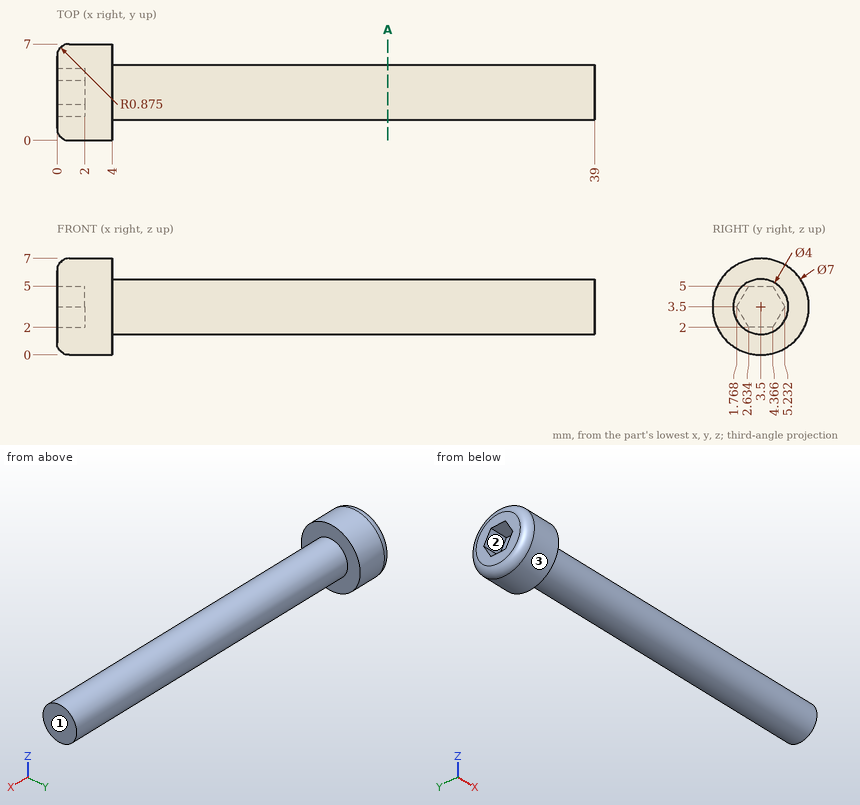
Here's the drawing with two shaded views (mm, measured from the low corner). I have some questions. Give positions to 0.01 mm unless a question says otherwise; leave off trailing zeros. Loops run counter-clockwise (first coordinate to the right, second up) from the corner with the lowest first, then second, coordinate; pieces in that order, holes last. Notation, with made-up numbers: M 32.5,-25.75 L 66.5,-25.75 A13 cw 66.5,-13.75 Z; hole C -14.5,-3.75 d5. An arc over 180 degrees is marked long. Use one line per item in the form item = value. Start each with the question number.
Q1. Will these pins go through, and if not, where does the flat tip stop? pin 1 Ø1.5 at (x, z) = (30, 1) entering from +Y; pin 2 Ø0.9 at (y, z) = (3, 3) entering from -X; pin 3 Ø2 at (x, z) = (26, 5.5) entering from +Y.
Q2. I need wall thicknesses on line 1 along Y through (x, z) = (17, 4.5); line 2 along Z through (x, y) = (36.5, 3.5); line 3 along X through (y, z) = (4.5, 1). Which ranges of each line are inside material? Lowest first, please.
Q3. If we section it at A-A (x = 24): Write out the boundary of the cut face in (y, z), then the cut area to 3 significant figures.
Q4. Thinking about a two-plate mould opening in Y: for the marked faces 1, 2 and 3, which applies, +Y half, -Y half, draft (parallel to the pull), parting line (faces both ways), or undercut?
Taken from the geometry:
q1.pin_1 = 4.47
q1.pin_2 = 2
q1.pin_3 = 5.23
q2.line_1 = 1.77 to 5.23
q2.line_2 = 1.5 to 5.5
q2.line_3 = 0 to 4
q3.outline = C 3.5,3.5 d4
q3.area = 12.6 mm^2
q4.face_1 = draft
q4.face_2 = undercut
q4.face_3 = parting line
